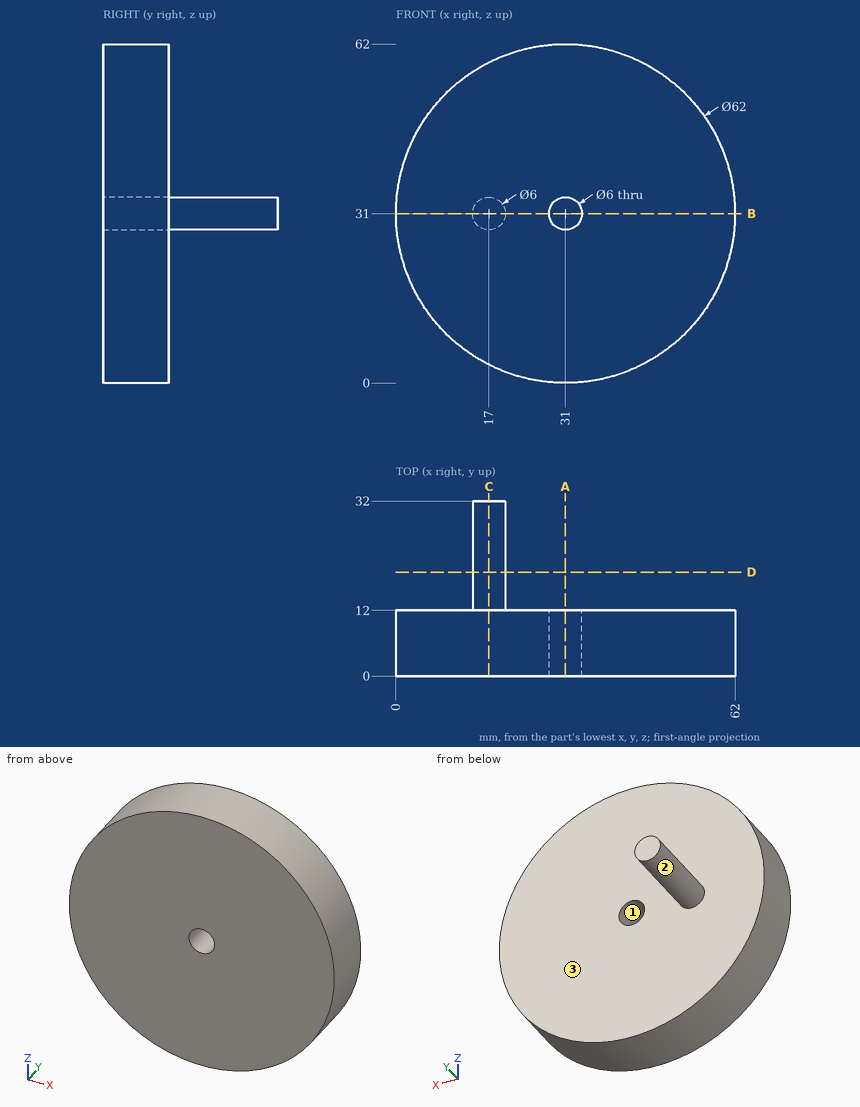
Geometry: see drawing. Coordinates: mm, zero at the bounding-box minimum. Give positions to 0.01 mm unless a question says otherwise; leave off trailing zeros. Loops run counter-clockwise (first coordinate to the right, second up) from the corner with the lowest first, then second, coordinate; pieces in that order, holes last. Notation, with made-up numbers: (21.25, 24) -> (80.25, 24) arc R7 ccw to (80.25, 35) -> close; hole circle Ø1 at (-18, 16). An arc over 180 degrees is marked (long way). Use one line per item in the form item = value.
Item 1: Section query A-A on x = 31. Output: boundary loops of the cut face in (y, z).
A:
outline = (0, 0) -> (12, 0) -> (12, 28) -> (0, 28) -> close; (0, 34) -> (12, 34) -> (12, 62) -> (0, 62) -> close
Item 2: Section query B-B on z = 31. Output: boundary loops of the cut face in (x, y), and give its area (3 significant figures).
A:
outline = (0, 0) -> (28, 0) -> (28, 12) -> (20, 12) -> (20, 32) -> (14, 32) -> (14, 12) -> (0, 12) -> close; (34, 0) -> (62, 0) -> (62, 12) -> (34, 12) -> close
area = 792 mm^2
Item 3: Line query: probe 1 along X at (y, z) = (8, 31); probe 2 along Y at (x, z) = (31.5, 54.5); probe 3 along Z at (x, y) = (16, 13.5). Output: solid intervals per line, ascending.
A:
probe_1 = 0 to 28, 34 to 62
probe_2 = 0 to 12
probe_3 = 28.17 to 33.83
Item 4: Section query C-C on x = 17. Output: boundary loops of the cut face in (y, z).
A:
outline = (0, 3.34) -> (12, 3.34) -> (12, 28) -> (32, 28) -> (32, 34) -> (12, 34) -> (12, 58.66) -> (0, 58.66) -> close
Item 5: Draft query along X for the marked faces 1, 2 and 3. Return one class per face: pulls with the +X half, pulls with the -X half, needs draft (parallel to the pull), parting line crosses it, or undercut.
A:
face_1 = undercut
face_2 = parting line crosses it
face_3 = needs draft
Item 6: Pin query (flat end, axial travel): P1, Ø1, axis at x = 19, y = 22, coming from the -Z side; P2, Ø4, axis at x = 44, z = 55.5, coming from the +Y side; P3, Ø8, axis at x = 36.5, y = 13, coming from the -Z side. Return the tip coordinate at first contact, or that it passes through.
A:
P1 = 28.4
P2 = 12
P3 = 0.04
Item 7: Section query D-D on y = 19. Output: boundary loops of the cut face in (x, z), and give its area (3 significant figures).
A:
outline = circle Ø6 at (17, 31)
area = 28.3 mm^2
